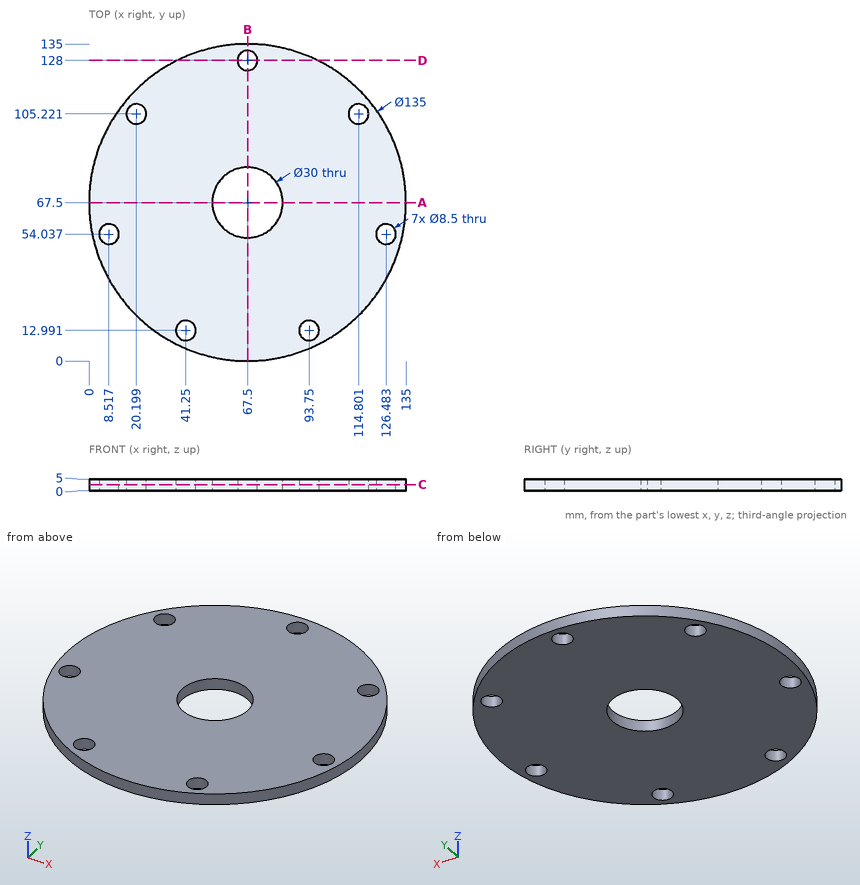
Source: three-view drawing plus pictorial views. Frame: mm from the lowest corner of the part. Give positions to 0.01 mm unless a question says otherwise; leave off trailing zeros. Loops run counter-clockwise (first coordinate to the right, second up) from the corner with the lowest first, then second, coordinate; pieces in that order, holes last. Notation, with made-up numbers: M -22.5,-36 L 1.5,-36 A22 ccw 1.5,-7 Z; hole C 65,68.5 d9. An arc over 180 degrees is marked long. Put each result on its own line as item: value.
Q1. Line query: probe 1 along Y at (x, z) = (68, 3.3); probe 2 along X at (y, z) = (68.5, 0.8); probe 3 along X at (y, z) = (106, 2.1) (1 decimal). Output: solid intervals per line, ascending. Write a range as [from, to].
Response values:
probe 1: y = [0, 52.51], [82.49, 123.78], [132.22, 135]
probe 2: x = [0.01, 52.53], [82.47, 134.99]
probe 3: x = [12.1, 16], [24.4, 110.6], [119, 122.9]
Q2. Section D-D (y = 128). Return the cut outline in (x, z).
Response values:
outline: M 37.57,0 L 63.25,0 L 63.25,5 L 37.57,5 Z; M 71.75,0 L 97.43,0 L 97.43,5 L 71.75,5 Z
Q3. Section A-A (y = 67.5). Return the cut outline in (x, z).
Response values:
outline: M 0,0 L 52.5,0 L 52.5,5 L 0,5 Z; M 82.5,0 L 135,0 L 135,5 L 82.5,5 Z
Q4. Section C-C (z = 2.6). Count the separate pieces of the cut face and the enclosed holes in it, and give its area (3 significant figures).
Response values:
separate pieces: 1
enclosed holes: 8
area: 13,200 mm²
Q5. Pin query (flat end, axial travel): P1, Ø2, axis at x = 77.5, z = 1.5, coming from the -Y side; P2, Ø5, axis at x = 67.5, y = 128, coming from the -Z side; P3, Ø3, axis at x = 71.5, z = 1, coming from the -Y side. Return the tip coordinate at first contact, or that it passes through.
Response values:
P1: stops at y = 0.6
P2: passes through
P3: stops at y = 0.05
Q6. Section B-B (x = 67.5). Return the cut outline in (y, z).
Response values:
outline: M 0,0 L 52.5,0 L 52.5,5 L 0,5 Z; M 82.5,0 L 123.75,0 L 123.75,5 L 82.5,5 Z; M 132.25,0 L 135,0 L 135,5 L 132.25,5 Z
